Design review of the part built by this model. Coordinates are the model's own, in mm. Face numbers are marked on the shaded views. A direction names the side the tool comes from. Coordinates: 2 decimals unless noted, no trailing zeros. Loops run counter-clockwise (first coordinate to the right, second up) from the corner with the lowest first, then second, coordinate; pieces in that order, holes last. Notation, with made-up numbers: (-4.75, 88) - (8.25, 88) arc R30 ccw to (8.25, 112) - close; hole circle Ø8 at (13.5, 62). An arc over 180 degrees is marked (long way). Return JSON: item names as keys, results as strings. Group by question number.
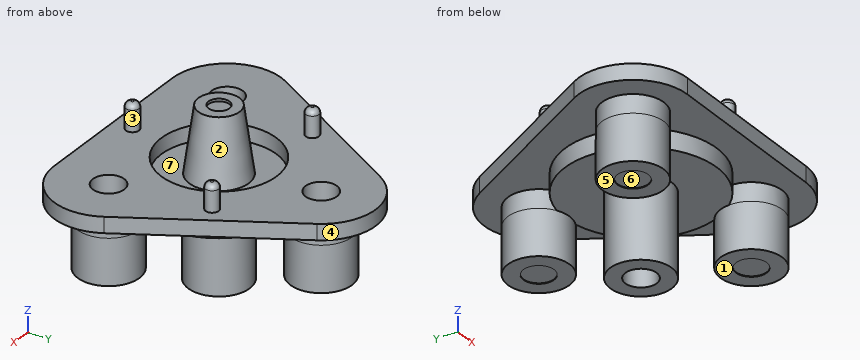
from build123d import *

# Parameters (mm, degrees)
BOSS_EXTRUDE1_DEPTH      = 1.524
SKETCH2_R                = 5.588
CUT_EXTRUDE1_DEPTH       = 1.4986
SKETCH3_R                = 2.8956
BOSS_EXTRUDE2_DEPTH      = 6.35
CHAMFER1_SIZE            = 6.35
CHAMFER1_SIZE_2          = 0.8924343
SKETCH4_R                = 1.016
CUT_EXTRUDE2_DEPTH       = 0.254
SKETCH5_R                = 7.366
BOSS_EXTRUDE3_DEPTH      = 1.778
BOSS_EXTRUDE4_DEPTH      = 1.778
CIRPATTERN1_COUNT        = 3
SKETCH7_R                = 2.9972
BOSS_EXTRUDE5_DEPTH      = 4.445
CIRPATTERN2_COUNT        = 3
SKETCH8_R                = 1.4859
CUT_EXTRUDE3_DEPTH       = 0.0508
CIRPATTERN3_COUNT        = 3
SKETCH9_R                = 2.9845
BOSS_EXTRUDE6_DEPTH      = 7.9248
CUT_EXTRUDE4_DEPTH       = 14.732
SKETCH11_R               = 1.524
CUT_EXTRUDE5_DEPTH       = 3.81
SKETCH16_R               = 1.524
CUT_EXTRUDE6_DEPTH       = 6.35
CIRPATTERN4_COUNT        = 3
SKETCH17_R               = 0.635
BOSS_EXTRUDE7_DEPTH      = 2.54
FILLET1_R                = 0.508
CIRPATTERN6_COUNT        = 3
FILLET1_OF_CIRPATTERN6_R = 0.508


with BuildPart() as part:
    # Sketch1 → Boss-Extrude1 (new body)
    with BuildSketch(Plane.XY):
        with BuildLine():
            Line((-4.591507335, 12.551273129), (-13.156663816, -2.315614668))
            ThreePointArc((-13.156663816, -2.315614668), (-13.153016231, -7.596706494), (-8.57884765, -10.2362))
            Line((-8.57884765, -10.2362), (8.57884765, -10.2362))
            ThreePointArc((8.57884765, -10.2362), (13.153016231, -7.596706494), (13.156663816, -2.315614668))
            Line((13.156663816, -2.315614668), (4.591507335, 12.551273129))
            ThreePointArc((4.591507335, 12.551273129), (0, 15.205000805), (-4.591507335, 12.551273129))
        make_face()
    extrude(amount=BOSS_EXTRUDE1_DEPTH)

    # Sketch2 → Cut-Extrude1 (cut)
    with BuildSketch(Plane.XY.offset(1.524)):
        Circle(SKETCH2_R)
    extrude(amount=-CUT_EXTRUDE1_DEPTH, mode=Mode.SUBTRACT)

    # Sketch3 → Boss-Extrude2 (add)
    with BuildSketch(Plane.XY.offset(0.0254)):
        Circle(SKETCH3_R)
    extrude(amount=BOSS_EXTRUDE2_DEPTH)

    # Chamfer1
    # the kernel refuses this chamfer: 6.35, 0.8924343 mm, written as the material it takes off along each edge
    with BuildSketch(Plane(origin=(0, 0, 6.3754), x_dir=(1, 0, 0), z_dir=(0, -1, 0))) as chamfer1_piece_1:
        Polygon((2.8956, -CHAMFER1_SIZE), (2.8956 - CHAMFER1_SIZE_2, 0), (2.8956, 0), align=None)
    revolve(axis=Axis((0, 0, 6.3754), (0, 0, 1)), mode=Mode.SUBTRACT)

    # Sketch4 → Cut-Extrude2 (cut)
    with BuildSketch(Plane.XY.offset(6.3754)):
        Circle(SKETCH4_R)
    extrude(amount=-CUT_EXTRUDE2_DEPTH, mode=Mode.SUBTRACT)

    # Sketch5 → Boss-Extrude3 (add)
    with BuildSketch(Plane(origin=(0, 0, 0), x_dir=(-1, 0, 0), z_dir=(0, 0, -1))):
        Circle(SKETCH5_R)
    extrude(amount=BOSS_EXTRUDE3_DEPTH)

    # Sketch6 → Boss-Extrude4 (add)
    with BuildSketch(Plane(origin=(0, 0, 0), x_dir=(-1, 0, 0), z_dir=(0, 0, -1))):
        with BuildLine():
            ThreePointArc((-1.366070827, 7.238218462), (0, 12.9032), (1.366070827, 7.238218462))
            ThreePointArc((1.366070827, 7.238218462), (0, 7.366), (-1.366070827, 7.238218462))
        make_face()
    boss_extrude4 = extrude(amount=BOSS_EXTRUDE4_DEPTH)

    # CirPattern1: Boss-Extrude4 ×3 about axis
    cirpattern1_axis = Axis((0, 0, 0), (0, 0, 1))
    for i in range(1, CIRPATTERN1_COUNT):
        add(boss_extrude4.rotate(cirpattern1_axis, i * 360 / CIRPATTERN1_COUNT))

    # Sketch7 → Boss-Extrude5 (add)
    with BuildSketch(Plane(origin=(0, 0, -1.778), x_dir=(-1, 0, 0), z_dir=(0, 0, -1))):
        with Locations(Location((0, 9.906, 0), (0, 0, 242.884717398))):
            Circle(SKETCH7_R)
    boss_extrude5 = extrude(amount=BOSS_EXTRUDE5_DEPTH)

    # CirPattern2: Boss-Extrude5 ×3 about axis
    cirpattern2_axis = Axis((0, 0, 0), (0, 0, 1))
    for i in range(1, CIRPATTERN2_COUNT):
        add(boss_extrude5.rotate(cirpattern2_axis, i * 360 / CIRPATTERN2_COUNT))

    # Sketch8 → Cut-Extrude3 (cut)
    with BuildSketch(Plane(origin=(0, 0, -6.223), x_dir=(-1, 0, 0), z_dir=(0, 0, -1))):
        with Locations((8.57884765, -4.953)):
            Circle(SKETCH8_R)
    cut_extrude3 = extrude(amount=-CUT_EXTRUDE3_DEPTH, mode=Mode.SUBTRACT)

    # CirPattern3: Cut-Extrude3 ×3 about axis
    cirpattern3_axis = Axis((0, 0, 0), (0, 0, 1))
    for i in range(1, CIRPATTERN3_COUNT):
        add(cut_extrude3.rotate(cirpattern3_axis, i * 360 / CIRPATTERN3_COUNT), mode=Mode.SUBTRACT)

    # Sketch9 → Boss-Extrude6 (add)
    with BuildSketch(Plane(origin=(0, 0, -1.778), x_dir=(-1, 0, 0), z_dir=(0, 0, -1))):
        Circle(SKETCH9_R)
    extrude(amount=BOSS_EXTRUDE6_DEPTH)

    # Sketch10 → Cut-Extrude4 (cut)
    with BuildSketch(Plane(origin=(0, 0, -9.7028), x_dir=(-1, 0, 0), z_dir=(0, 0, -1))):
        Polygon((-1.466469684, 0), (-0.733234842, -1.27), (0.733234842, -1.27), (1.466469684, 0), (0.733234842, 1.27), (-0.733234842, 1.27), align=None)
    extrude(amount=-CUT_EXTRUDE4_DEPTH, mode=Mode.SUBTRACT)

    # Sketch11 → Cut-Extrude5 (cut)
    with BuildSketch(Plane(origin=(0, 0, -9.7028), x_dir=(-1, 0, 0), z_dir=(0, 0, -1))):
        Circle(SKETCH11_R)
    extrude(amount=-CUT_EXTRUDE5_DEPTH, mode=Mode.SUBTRACT)

    # Sketch16 → Cut-Extrude6 (cut)
    with BuildSketch(Plane.XY.offset(1.524)):
        with Locations((-8.57884765, -4.953)):
            Circle(SKETCH16_R)
    cut_extrude6 = extrude(amount=-CUT_EXTRUDE6_DEPTH, mode=Mode.SUBTRACT)

    # CirPattern4: Cut-Extrude6 ×3 about axis
    cirpattern4_axis = Axis((0, 0, 0), (0, 0, 1))
    for i in range(1, CIRPATTERN4_COUNT):
        add(cut_extrude6.rotate(cirpattern4_axis, i * 360 / CIRPATTERN4_COUNT), mode=Mode.SUBTRACT)

    # Sketch17 → Boss-Extrude7 (add)
    with BuildSketch(Plane.XY.offset(1.524)):
        with Locations(Location((0, -8.382, 0), (0, 0, 180))):
            Circle(SKETCH17_R)
    boss_extrude7 = extrude(amount=BOSS_EXTRUDE7_DEPTH)

    # Fillet1
    fillet1_edges = [part.edges().sort_by_distance(p)[0] for p in [
        (0.635, -8.382, 4.064),
    ]]
    fillet(fillet1_edges, radius=FILLET1_R)

    # CirPattern6: Boss-Extrude7 ×3 about axis
    cirpattern6_axis = Axis((0, 0, 0), (0, 0, 1))
    for i in range(1, CIRPATTERN6_COUNT):
        add(boss_extrude7.rotate(cirpattern6_axis, i * 360 / CIRPATTERN6_COUNT))

    # Fillet1 of CirPattern6
    fillet1_of_cirpattern6_edges = [part.edges().sort_by_distance(p)[0] for p in [
        (6.941524935, 4.740926131, 4.064),
        (-7.576524935, 3.641073869, 4.064),
    ]]
    fillet(fillet1_of_cirpattern6_edges, radius=FILLET1_OF_CIRPATTERN6_R)


solid = part.part
Item 1: To check wall thickness, follow line 1 (Y direction, x = 0, z = -3.5); line 2 (X direction, y = -2.75, z = -4.5); line 3 (Z direction, x = -4.25, y = -8). State the ranges of each line that lie inside material, in increasing order. Write a range as from..to.
Item 2: Add section B-B (z = -1.25). State the section outline as (x, y) points.
Item 3: Add section D-D (z = -7). State the section outline as (x, y) points.
Item 4: For the marked faces 4, 5, 6 and 7, list the 3-axis set-ups (+Z, -Z, +X, -X, +Y, -Y) from which the entire face can be reached by the end or side of a thin tool; tool diameter is ignored.
Item 5: Add section A-A (z = -5.25). State the section outline as (x, y) points.
Item 6: For P1, Ø0.6, axis at x = 0, y = 0, coming from the +Z side; P2, Ø5, axis at y = -2, z = -2, coming from the +X side; P3, Ø1.6, axis at x = 0, z = -2.5, coming from the +Y side; P4, Ø2, axis at y = -3.5, z = 4, coming from the -X side, all flat-tipped, find the tip position at first contact; note any pin that passes through.
Item 7: Add section C-C (x = 10.5). State the section outline as (y, z) points.
Item 8: Draft analysis for pull direction X (two halves, no side actions). For the marked faces 1, 2 and 3, state which applies: pulls with the +X half, pulls with the -X half, needs draft (parallel to the pull), parting line crosses it, or undercut.
Answers below:
{
 "1": {"line 1": "y = -2.98..-1.27, 1.27..2.98, 6.91..8.38, 11.43..12.9", "line 2": "x = -10.61..-6.55, -1.16..1.16, 6.55..10.61", "line 3": "z = 0..1.52"},
 "2": {"outline": "(-6.95, -2.44) arc R3 ccw (long way) to (-5.59, -4.8) arc R7.37 ccw to (5.59, -4.8) arc R3 ccw (long way) to (6.95, -2.44) arc R7.37 ccw to (1.37, 7.24) arc R3 ccw (long way) to (-1.37, 7.24) arc R7.37 ccw to start; hole circle Ø3.05 at (-8.58, -4.95); hole circle Ø3.05 at (0, 9.91); hole (-1.47, 0) - (-0.73, -1.27) - (0.73, -1.27) - (1.47, 0) - (0.73, 1.27) - (-0.73, 1.27) - close; hole circle Ø3.05 at (8.58, -4.95)"},
 "3": {"outline": "circle Ø5.97 at (0, 0); hole circle Ø3.05 at (0, 0)"},
 "4": {"face 4": "+Z, -Z, +Y", "face 5": "-Z, -X, +Y, -Y", "face 6": "-Z", "face 7": "+Z"},
 "5": {"outline": "circle Ø5.99 at (-8.58, -4.95); circle Ø5.99 at (0, 9.91); circle Ø5.97 at (0, 0); circle Ø5.99 at (8.58, -4.95); hole (-1.47, 0) - (-0.73, -1.27) - (0.73, -1.27) - (1.47, 0) - (0.73, 1.27) - (-0.73, 1.27) - close"},
 "6": {"P1": "stops at z = 6.12", "P2": "stops at x = 13.66", "P3": "stops at y = 12.9", "P4": "passes through"},
 "7": {"outline": "(-9.87, 0) - (-7.25, 0) - (-7.25, -6.22) - (-2.65, -6.22) - (-2.65, 0) - (2.3, 0) - (2.3, 1.52) - (-9.87, 1.52) - close"},
 "8": {"face 1": "needs draft", "face 2": "undercut", "face 3": "parting line crosses it"}
}
